Design review of the part built by this model. Coordinates are the model's own, in mm. Face numbers are marked on the shaded views. A direction names the side the tool comes from. Round coordinates to 2 decimals unless told otherwise and drop trailing zeros. Loops run counter-clockwise (first coordinate to the right, second up) from the corner with the lowest first, then second, coordinate; pieces in that order, holes last. Notation, with made-up numbers: (14, 70) -> (57, 70) arc R23 ccw to (57, 83) -> close; hole circle Ø3 at (-38.75, -1). An arc over 180 degrees is marked (long way). Use a Markdown table: item, result. Add a question column.
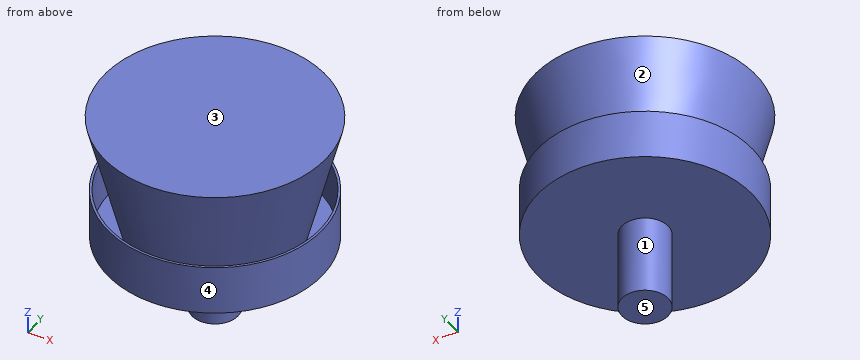
Autodesk Inventor part; units mm, degrees
ref_plane "Work Plane4" through (-298.3836, 2.4745, -42.75) normal (0, 0, -1) x (0, 1, 0)
ref_plane "YZ Plane" through (0, 0, 0) normal (1, 0, 0) x (0, 1, 0)
ref_plane "XY Plane" through (0, 0, 0) normal (0, 0, 1) x (1, 0, 0)
ref_plane "Work Plane1" through (0, 0, -0.5) normal (0, 0, -1) x (-1, 0, 0)
sketch "Sketch1" plane through (0, 0, -0.5) normal (0, 0, -1) x (-1, 0, 0)
  line L0 (134.0347, 37.6976) -> (134.0347, -12.3024)
  line L1 (134.0347, 37.6976) -> (30.0097, 37.6976)
  line L2 (30.0097, 37.6976) -> (30.0097, 128.6976)
  line L3 (-19.9903, 128.6976) -> (30.0097, 128.6976)
  line L4 (-19.9903, 128.6976) -> (-19.9903, 37.6976)
  line L5 (-19.9903, 37.6976) -> (-140.9903, 37.6976)
  line L6 (-140.9903, -12.3024) -> (-140.9903, 37.6976)
  line L7 (-140.9903, -12.3024) -> (-19.9903, -12.3024)
  line L8 (-19.9903, -12.3024) -> (-19.9903, -146.3274)
  line L9 (30.0097, -146.3274) -> (-19.9903, -146.3274)
  line L10 (30.0097, -146.3274) -> (30.0097, -12.3024)
  line L11 (30.0097, -12.3024) -> (134.0347, -12.3024)
  line L12 (-19.9903, 37.6976) -> (30.0097, -12.3024) construction
  line L13 (30.0097, 37.6976) -> (-19.9903, -12.3024) construction
  circle A0 centre (5.0097, 12.6976) radius 20
  point P0 (0, 0)
  dimension "d0" = 40
extrude "Extrusion1" add sketch "Sketch1" against normal blind 25.75 contours A0
sketch "Sketch2" plane through (-5.0097, 12.6976, 25.25) normal (0, 0, 1) x (1, 0, 0)
  circle A0 centre (0, 0) radius 92.639
  point P0 (5.0097, -12.6976)
extrude "Extrusion2" add sketch "Sketch2" along normal blind 42.75
shell "Shell1" thickness 2 removed faces 1 at (-24.2409, 34.4376, 68)
ref_plane "Work Plane3" through (-5.0097, 12.6976, -0.5) normal (0, 1, 0) x (-1, 0, 0)
ref_plane "Work Plane2" through (-5.0097, -7.3024, -0.5) normal (0, 1, 0) x (-1, 0, 0)
sketch "Sketch3" plane through (-5.0097, 12.6976, -0.5) normal (0, 1, 0) x (-1, 0, 0)
  line L0 (18, 27.75) -> (-18, 27.75)
  line L1 (0, 27.75) -> (-68, 27.75)
  line L2 (90.639, 27.75) -> (-90.639, 27.75)
  line L3 (-68, 27.75) -> (-95.6652, 136.8622)
  line L4 (-95.6652, 136.8622) -> (0, 136.8622)
  line L5 (0, 136.8622) -> (0, 27.75)
  point P0 (-5.0097, 0.5)
  dimension "d8" = 95.6652
  dimension "d9" = 68
revolve "Revolution1" add sketch "Sketch3" angle 360 about axis through (-5.0097, 12.6976, 136.3622) along (0, 0, -1)
ref_plane "Work Plane4" through (-298.3836, 2.4745, -42.75) normal (0, 0, -1) x (0, 1, 0)
sketch "Sketch4" plane through (-5.0097, 12.6976, -0.5) normal (0, 0, -1) x (-1, 0, 0)
  circle A0 centre (0, 0) radius 20
  point P0 (-5.0097, -12.6976)
extrude "Extrusion3" add sketch "Sketch4" along normal up to surface (42.25 mm away)
properties part number "BRUSH1"
1. Insertion check: P1, Ø4, axis at x = 64, y = 52.5, coming from the -Z side; P2, Ø1.5, axis at y = 38.5, z = 92.5, coming from the +X side; P3, Ø12, axis at x = -20, z = -13.5, coming from the -Y side. Each pin has a flat end and moves straight along its axis. Give the tip position at first contact, or say it passes through.
2. For the marked faces 4 and 5, list the 3-axis set-ups (+Z, -Z, +X, -X, +Y, -Y) from which the entire face can be reached by the end or side of a thin tool; tool diameter is ignored.
3. Mouldability with a two-part tool opening along X and no side actions: class the marked faces 1, 2 and 3 as +X half, -X half, draft (parallel to the pull), parting line (faces both ways), or undercut.
4. Consider section C-C on z = 92.5. State the section outline as (x, y) points, plus the area to 3 significant figures.
5. Consider section B-B on z = 112.5. State the section outline as (x, y) points.
6. To check wall thickness, follow probe 1 along Y at (x, z) = (54.5, 58.5); probe 2 along Y at (x, z) = (61, 49); probe 3 along X at (y, z) = (16.5, 16). State the ranges of each line that lie inside material, in increasing order. Write a range as from..to.
7. Consider section A-A on z = 37. State the section outline as (x, y) points, plus the area to 3 significant figures.
Verdict:
| question | item | result |
|---|---|---|
| 1 | P1 | stops at z = 25.25 |
| 1 | P2 | stops at x = 75.81 |
| 1 | P3 | stops at y = -5.17 |
| 2 | face 4 | -Z |
| 2 | face 5 | -Z, +X, -X, +Y, -Y |
| 3 | face 1 | parting line |
| 3 | face 2 | undercut |
| 3 | face 3 | draft |
| 4 | outline | circle Ø169.09 at (-5.01, 12.7) |
| 4 | area | 22,500 mm² |
| 5 | outline | circle Ø179.23 at (-5.01, 12.7) |
| 6 | probe 1 | y = -58.3..-55.67, -34.45..59.85, 81.06..83.69 |
| 6 | probe 2 | y = -52.3..-49.42, -19.66..45.06, 74.81..77.7 |
| 6 | probe 3 | x = -24.64..-22.6, 12.58..14.63 |
| 7 | outline | circle Ø185.28 at (-5.01, 12.7); circle Ø140.94 at (-5.01, 12.7); hole circle Ø181.28 at (-5.01, 12.7) |
| 7 | area | 16,800 mm² |
